Could you check a few things on this model? Use its own coordinates, in mm. A direction names the side the tool comes from. Coordinates: 2 decimals unless noted, no trailing zeros. Write each loop counter-clockwise with the first axis right and the second up, starting at its lowest first coordinate (ties: lowest second). Pieces come first, ordered by that corner, then holes.
```python
from build123d import *

# Parameters (mm, degrees)
F0_W     = 42.5
F0_H     = 16.5
F1_DEPTH = 1.6
F2_W     = 19.383784
F2_H     = 11.430836
F2_W_2   = 3.613464
F2_H_2   = 13.885942
F3_DEPTH = 2
F4_W     = 1.4
F4_H     = 12
F5_DEPTH = 3


with BuildPart() as f1:
    # F0 (on Top) → F1 (new body)
    with BuildSketch(Plane.XY):
        Rectangle(F0_W, F0_H)
    extrude(amount=F1_DEPTH)

    # F2 (on face) → F3 (join)
    with BuildSketch(Plane.XY.offset(1.6)):
        Rectangle(F2_W, F2_H)
        with Locations((15.997825, 0)):
            Rectangle(F2_W_2, F2_H_2)
    extrude(amount=F3_DEPTH)

    # F4 (on face) → F5 (join)
    with BuildSketch(Plane(origin=(0, 0, 0), x_dir=(1, 0, 0), z_dir=(0, 0, -1))):
        with Locations((-18.55, 0)):
            Rectangle(F4_W, F4_H)
    extrude(amount=F5_DEPTH)


solid = f1.part
```
Item 1: If I drill on line 1 along X through (y, z) = (-0.25, -2); line 2 along Z through (x, y) = (19, 4.75); line 3 along Z through (x, y) = (0, -5.5), over which ranges is the centre line in solid material (lowest first)?
Item 2: I want a section at D-D, the plane y = 3. List the corners of the cut face in (x, z) for me, then the cut area to 3 significant figures.
Item 3: I want a section at B-B, the plane y = 6.5. List the corners of the cut face in (x, z) for me, then the cut area to 3 significant figures.
Item 4: I want a section at A-A, the plane x = -8. List the corners of the cut face in (y, z) for me.
Item 5: Will these pins go through, and if not, where does the flat tip stop? pin 1 Ø0.7 at (x, z) = (-18, -1.5) entering from +Y; pin 2 Ø1.6 at (y, z) = (-1.5, 3) entering from +X; pin 3 Ø1 at (x, y) = (14.5, 3) entering from -Z.
Item 6: I want a section at C-C, the plane z = -2. List the corners of the cut face in (x, y) for me.
Item 7: If we mould it in two halves opening along X, with no side actions, what happens to faces 5 (the flat face through (-17.85, 0, -1)), 6 (the flat face through (9.692, 0, 3)), 7 (the flat face through (16, 0, 3.6))? For each: released by +X, released by -X, zero draft, split by the parting line, or undercut.
Item 8: Which directions (+Z, -Z, +X, -X, +Y, -Y) give clear straight access to the entire face, cutting with the end or side of a thin tool? Please do faces 1 (the flat face through (16, 6.943, 3)), 2 (the flat face through (-19, -6, -1)), 3 (the flat face through (17.805, 0, 3)), 4 (the flat face through (-19, 6, -1)).
Taken from the geometry:
1. line 1: x = -19.25 to -17.85
1. line 2: z = 0 to 1.6
1. line 3: z = 0 to 3.6
2. outline: (-21.25, 0) - (-19.25, 0) - (-19.25, -3) - (-17.85, -3) - (-17.85, 0) - (21.25, 0) - (21.25, 1.6) - (17.8, 1.6) - (17.8, 3.6) - (14.19, 3.6) - (14.19, 1.6) - (9.69, 1.6) - (9.69, 3.6) - (-9.69, 3.6) - (-9.69, 1.6) - (-21.25, 1.6) - close
2. area: 118 mm2
3. outline: (-21.25, 0) - (21.25, 0) - (21.25, 1.6) - (17.8, 1.6) - (17.8, 3.6) - (14.19, 3.6) - (14.19, 1.6) - (-21.25, 1.6) - close
3. area: 75.2 mm2
4. outline: (-8.25, 0) - (8.25, 0) - (8.25, 1.6) - (5.72, 1.6) - (5.72, 3.6) - (-5.72, 3.6) - (-5.72, 1.6) - (-8.25, 1.6) - close
5. pin 1: stops at y = 6
5. pin 2: stops at x = 17.8
5. pin 3: stops at z = 0
6. outline: (-19.25, -6) - (-17.85, -6) - (-17.85, 6) - (-19.25, 6) - close
7. face 5: released by +X
7. face 6: undercut
7. face 7: zero draft
8. face 1: +Z, +X, -X, +Y
8. face 2: -Z, +X, -X, -Y
8. face 3: +Z, +X, +Y, -Y
8. face 4: -Z, +X, -X, +Y
